Geometry check sheet. Reference: the model listing, model coordinates, mm. Face numbers are marked on the shaded views. A direction names the side the tool comes from. Coordinates: 2 decimals unless noted, no trailing zeros. Write each loop counter-clockwise with the first axis right and the second up, starting at its lowest first coordinate (ties: lowest second). Pieces come first, ordered by that corner, then holes. Notation, with made-up numbers: M 63,-27.75 L 104,-27.75 A22 ccw 104,-21.75 Z; hole C 37,44 d1. An arc over 180 degrees is marked long. Put each result on its own line as item: value. Start each with the question number.
1) Cross-section at B-B on y = 13.25. Record the cut outline in (x, z).
2) Cross-section at C-C on x = -1.5. Record the cut outline in (y, z).
3) Scan lines: line 1 along Z through (x, y) = (7.85, 18); line 2 along Z through (x, y) = (-5.5, 16.25); line 3 along Z through (x, y) = (-7, 11.5). Record each from-to range of solid material in increasing order.
4) Gauge pin test, flat ends, axial feed: pin 1 (8 mm diameter, centred on y = 13, z = -2.5, fed in from +X); pin 2 (1.9 mm diameter, centred on x = 7, z = 13.5, fed in from +Y); pin 3 (3.5 mm diameter, centred on x = 15.5, z = 13.5, fed in from -Y). Record the tip position at first contact, or that the pin passes through.
5) Mould release check, pull along Z, two halves, no side actions. Record for the marked faces 1, 2 and 3: released by +Z, released by -Z, zero draft, split by the parting line, or undercut.
6) Set-up check for the marked faces 4, 5 and 6: record each of +Z, -Z, +X, -X, +Y, -Y from which the full face is reachable in a straight line by a thin tool's end or side.
7) Cross-section at D-D on z = -13.5. Record the cut outline in (x, y), plus the area to 3 significant figures.
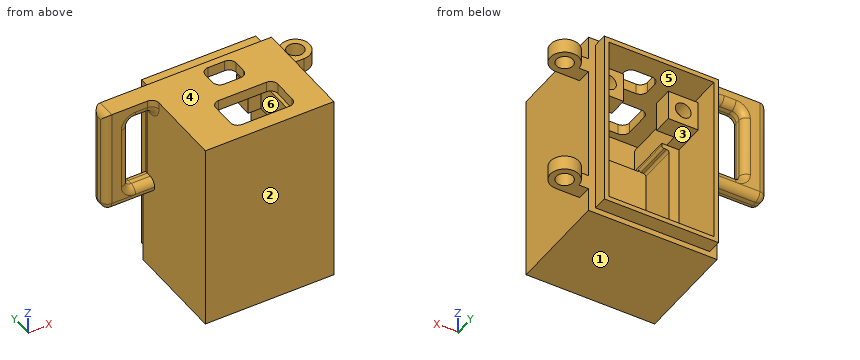
from build123d import *

# Parameters (mm, degrees)
SKETCH2_W                 = 27
SKETCH2_H                 = 40
BOSS_EXTRUDE1_DEPTH       = 1.5
SKETCH3_W                 = 27
SKETCH3_H                 = 40
SKETCH3_W_2               = 22
SKETCH3_H_2               = 35.62
BOSS_EXTRUDE2_DEPTH       = 20
SKETCH4_R                 = 1.75
BOSS_EXTRUDE3_DEPTH       = 40
BOSS_EXTRUDE4_DEPTH       = 11
SKETCH8_W                 = 17.78
SKETCH8_H                 = 20.7
BOSS_EXTRUDE5_DEPTH       = 3
FILLET1_R                 = 0.5
SKETCH9_W                 = 3.61
SKETCH9_H                 = 6.3
BOSS_EXTRUDE6_DEPTH       = 13.64
SKETCH10_W                = 6.3
SKETCH10_H                = 6.3
BOSS_EXTRUDE7_DEPTH       = 4
F_3_0MM_DOWEL_HOLE2_D     = 3.3
F_3_0MM_DOWEL_HOLE2_DEPTH = 2.8
F_3_0MM_DOWEL_HOLE2_TIP   = 0.991420021
CUT_EXTRUDE1_REACH        = 53.599
SKETCH13_W                = 13
SKETCH13_H                = 8
FILLET2_R                 = 1.5
CUT_EXTRUDE2_REACH        = 53.599
SKETCH14_W                = 6.5
SKETCH14_H                = 5.5
FILLET3_R                 = 1.5
SKETCH15_W                = 24
SKETCH15_H                = 37.62
SKETCH15_W_2              = 22
SKETCH15_H_2              = 35.62
BOSS_EXTRUDE8_DEPTH       = 3
BOSS_EXTRUDE9_DEPTH       = 4
FILLET4_R                 = 1.5
SKETCH17_W                = 5
SKETCH17_H                = 29.710811322
SKETCH17_H_2              = 26.502201667
SKETCH17_W_2              = 24
SKETCH17_H_3              = 26.060216056
CUT_EXTRUDE3_DEPTH        = 50.056090346


with BuildPart() as part:
    # Sketch2 → Boss-Extrude1 (new body)
    with BuildSketch(Plane(origin=(0, 0, 0), x_dir=(1, 0, 0), z_dir=(0, 1, 0))):
        Rectangle(SKETCH2_W, SKETCH2_H)
    extrude(amount=BOSS_EXTRUDE1_DEPTH)

    # Sketch3 → Boss-Extrude2 (add)
    with BuildSketch(Plane(origin=(0, 1.5, 0), x_dir=(1, 0, 0), z_dir=(0, 1, 0))):
        Rectangle(SKETCH3_W, SKETCH3_H)
        Rectangle(SKETCH3_W_2, SKETCH3_H_2, mode=Mode.SUBTRACT)
    extrude(amount=BOSS_EXTRUDE2_DEPTH)

    # Sketch4 → Boss-Extrude3 (add, through all)
    with BuildSketch(Plane.XY.offset(20)):
        with BuildLine():
            Line((15.5, 21.5), (13.5, 21.5))
            Line((13.5, 21.5), (13.5, 18.5))
            Line((13.5, 18.5), (18.5, 18.5))
            ThreePointArc((18.5, 18.5), (20.621320344, 23.621320344), (15.5, 21.5))
        make_face()
        with Locations((18.5, 21.5)):
            Circle(SKETCH4_R, mode=Mode.SUBTRACT)
    extrude(amount=-BOSS_EXTRUDE3_DEPTH)

    # Sketch6 → Boss-Extrude4 (add)
    with BuildSketch(Plane(origin=(0, 1.5, 0), x_dir=(1, 0, 0), z_dir=(0, 1, 0))):
        Polygon((8.89, -10.51), (7.39, -10.51), (7.39, -9.51), (8.89, -9.51), (8.89, 11.19), (7.39, 11.19), (7.39, 12.19), (8.89, 12.19), (11, 12.19), (11, -10.51), align=None)
        Polygon((-8.89, -10.51), (-11, -10.51), (-11, 12.19), (-8.89, 12.19), (-7.39, 12.19), (-7.39, 11.19), (-8.89, 11.19), (-8.89, -9.51), (-7.39, -9.51), (-7.39, -10.51), align=None)
    extrude(amount=BOSS_EXTRUDE4_DEPTH)

    # Sketch8 → Boss-Extrude5 (add)
    with BuildSketch(Plane(origin=(0, 1.5, 0), x_dir=(1, 0, 0), z_dir=(0, 1, 0))):
        with Locations((0, 0.84)):
            Rectangle(SKETCH8_W, SKETCH8_H)
    extrude(amount=BOSS_EXTRUDE5_DEPTH)

    # Fillet1
    fillet1_edges = [part.edges().sort_by_distance(p)[0] for p in [
        (7.39, 8.5, 9.51),
        (7.39, 8.5, -11.19),
        (8.89, 8.5, -11.19),
        (8.89, 8.5, 9.51),
        (-7.39, 8.5, 9.51),
        (-8.89, 8.5, 9.51),
        (-8.89, 8.5, -11.19),
        (-7.39, 8.5, -11.19),
    ]]
    fillet(fillet1_edges, radius=FILLET1_R)

    # Sketch9 → Boss-Extrude6 (add)
    with BuildSketch(Plane(origin=(0, 1.5, 0), x_dir=(1, 0, 0), z_dir=(0, 1, 0))):
        with Locations((-10.195, -13.66)):
            Rectangle(SKETCH9_W, SKETCH9_H)
        with Locations((9.195, -13.66)):
            Rectangle(SKETCH9_W, SKETCH9_H)
    extrude(amount=BOSS_EXTRUDE6_DEPTH)

    # Sketch10 → Boss-Extrude7 (add)
    with BuildSketch(Plane(origin=(0, 15.14, 0), x_dir=(1, 0, 0), z_dir=(0, 1, 0))):
        with Locations((-7.85, -13.66)):
            Rectangle(SKETCH10_W, SKETCH10_H)
        with Locations((7.85, -13.66)):
            Rectangle(SKETCH10_W, SKETCH10_H)
    extrude(amount=BOSS_EXTRUDE7_DEPTH)

    # Ø3.0mm Dowel Hole2
    with Locations(Plane(origin=(0, 19.14, 0), x_dir=(1, 0, 0), z_dir=(0, 1, 0))):
        with Locations((7.85, -13.66), (-7.85, -13.66)):
            Hole(F_3_0MM_DOWEL_HOLE2_D / 2, depth=F_3_0MM_DOWEL_HOLE2_DEPTH)
            with Locations((0, 0, -(F_3_0MM_DOWEL_HOLE2_DEPTH + F_3_0MM_DOWEL_HOLE2_TIP / 2))):  # 118° drill point
                Cone(0, F_3_0MM_DOWEL_HOLE2_D / 2, F_3_0MM_DOWEL_HOLE2_TIP, mode=Mode.SUBTRACT)

    # Sketch13 → Cut-Extrude1 (cut, up to next)
    with BuildSketch(Plane.XY.offset(20), mode=Mode.PRIVATE) as cut_extrude1_sk1:
        with Locations((1, 7)):
            Rectangle(SKETCH13_W, SKETCH13_H)
    cut_extrude1_tool1 = extrude(cut_extrude1_sk1.sketch, amount=-CUT_EXTRUDE1_REACH, mode=Mode.PRIVATE) & part.part
    add(cut_extrude1_tool1.solids().sort_by_distance((1, 7, 20))[0], mode=Mode.SUBTRACT)

    # Fillet2
    fillet2_edges = [part.edges().sort_by_distance(p)[0] for p in [
        (7.5, 3, 18.905),
        (7.5, 11, 18.905),
        (-5.5, 11, 18.905),
        (-5.5, 3, 18.905),
    ]]
    fillet(fillet2_edges, radius=FILLET2_R)

    # Sketch14 → Cut-Extrude2 (cut, up to next)
    with BuildSketch(Plane.XY.offset(20), mode=Mode.PRIVATE) as cut_extrude2_sk1:
        with Locations((1, 17.25)):
            Rectangle(SKETCH14_W, SKETCH14_H)
    cut_extrude2_tool1 = extrude(cut_extrude2_sk1.sketch, amount=-CUT_EXTRUDE2_REACH, mode=Mode.PRIVATE) & part.part
    add(cut_extrude2_tool1.solids().sort_by_distance((1, 17.25, 20))[0], mode=Mode.SUBTRACT)

    # Fillet3
    fillet3_edges = [part.edges().sort_by_distance(p)[0] for p in [
        (4.25, 14.5, 18.905),
        (4.25, 20, 18.905),
        (-2.25, 20, 18.905),
        (-2.25, 14.5, 18.905),
    ]]
    fillet(fillet3_edges, radius=FILLET3_R)

    # Sketch15 → Boss-Extrude8 (add)
    with BuildSketch(Plane(origin=(0, 21.5, 0), x_dir=(1, 0, 0), z_dir=(0, 1, 0))):
        Rectangle(SKETCH15_W, SKETCH15_H)
        Rectangle(SKETCH15_W_2, SKETCH15_H_2, mode=Mode.SUBTRACT)
    extrude(amount=BOSS_EXTRUDE8_DEPTH)

    # Sketch16 → Boss-Extrude9 (add)
    with BuildSketch(Plane(origin=(0, 21.5, 0), x_dir=(1, 0, 0), z_dir=(0, 1, 0))):
        Polygon((-13.5, -17), (-13.5, -20), (-24, -20), (-24, 2), (-13.5, 2), (-13.5, -1), (-19, -1), (-19, -17), align=None)
    extrude(amount=-BOSS_EXTRUDE9_DEPTH)

    # Fillet4
    fillet4_edges = [part.edges().sort_by_distance(p)[0] for p in [
        (-13.5, 17.5, 18.5),
        (-13.5, 21.5, 9),
        (-16.25, 17.5, 1),
        (-16.25, 17.5, 17),
        (-13.5, 19.5, 17),
        (-19, 17.5, 9),
        (-19, 19.5, 1),
        (-19, 19.5, 17),
        (-16.25, 21.5, 17),
        (-19, 21.5, 9),
        (-16.25, 21.5, 1),
        (-18.75, 17.5, -2),
        (-18.75, 21.5, -2),
        (-24, 19.5, 20),
        (-24, 21.5, 9),
        (-24, 17.5, 9),
        (-24, 19.5, -2),
    ]]
    fillet(fillet4_edges, radius=FILLET4_R - 0.0001)  # a hair under: the kernel refuses the full size

    # Sketch17 → Cut-Extrude3 (cut, through all)
    with BuildSketch(Plane(origin=(13.5, 0, 0), x_dir=(0, 0, -1), z_dir=(1, 0, 0))):
        with Locations((-17.5, 14.855405661)):
            Rectangle(SKETCH17_W, SKETCH17_H)
        with Locations((17.5, 13.251100834)):
            Rectangle(SKETCH17_W, SKETCH17_H_2)
        with Locations((0, 13.030108028)):
            Rectangle(SKETCH17_W_2, SKETCH17_H_3)
    extrude(amount=CUT_EXTRUDE3_DEPTH, mode=Mode.SUBTRACT)


solid = part.part
Answer key:
1. outline: M -13.5,-20 L 13.5,-20 L 13.5,20 L -13.5,20 Z; hole M -11,-17.81 L 11,-17.81 L 11,10.51 L 7.39,10.51 L 7.39,16.81 L 11,16.81 L 11,17.81 L -11,17.81 L -11,16.81 L -8.39,16.81 L -8.39,10.51 L -11,10.51 Z
2. outline: M 0,-20 L 21.5,-20 L 21.5,-18.81 L 24.5,-18.81 L 24.5,-17.81 L 1.5,-17.81 L 1.5,-11.19 L 4.5,-11.19 L 4.5,9.51 L 1.5,9.51 L 1.5,17.81 L 3,17.81 L 3,20 L 0,20 Z; M 11,17.81 L 14.7,17.81 L 14.7,20 L 11,20 Z; M 19.8,17.81 L 24.5,17.81 L 24.5,18.81 L 21.5,18.81 L 21.5,20 L 19.8,20 Z
3. line 1: z = -20 to -17.81, 10.51 to 12.01, 15.31 to 16.81, 17.81 to 20
3. line 2: z = -20 to -17.81, 10.51 to 16.81, 17.81 to 20
3. line 3: z = -20 to -17.81, 17.81 to 20
4. pin 1: stops at x = 13.5
4. pin 2: stops at y = 19.14
4. pin 3: stops at y = 18.5
5. face 1: released by -Z
5. face 2: zero draft
5. face 3: undercut
6. face 4: +Z, +X, -X, +Y, -Y
6. face 5: +Y
6. face 6: none
7. outline: M -13.5,0 L 13.5,0 L 13.5,18.5 L 18.5,18.5 A3 ccw long 15.5,21.5 L 12,21.5 L 12,24.5 L 11,24.5 L 11,1.5 L -11,1.5 L -11,24.5 L -12,24.5 L -12,21.5 L -13.5,21.5 Z; hole C 18.5,21.5 d3.5
7. area: 173 mm²
